```python
from build123d import *

# Parameters (mm, degrees)
F1_DEPTH = 25
F2_DEPTH = 25
F3_DEPTH = 25
F4_DEPTH = 25
F5_DEPTH = 25
F6_DEPTH = 25


with BuildPart() as f1:
    # F0 (on Top) → F1 (new body)
    with BuildSketch(Plane.XY):
        Polygon((264.877629, 90.833528), (-135.122371, 90.833528), (-18.141241, -204.166472), (181.858759, -204.166472), align=None)
    extrude(amount=F1_DEPTH)

    # F0 (on Top) → F2 (join)
    with BuildSketch(Plane.XY):
        Polygon((264.877629, 90.833528), (-135.122371, 90.833528), (-18.141241, -204.166472), (181.858759, -204.166472), align=None)
    extrude(amount=F2_DEPTH)

    # F0 (on Top) → F3 (join)
    with BuildSketch(Plane.XY):
        Polygon((264.877629, 90.833528), (-135.122371, 90.833528), (-18.141241, -204.166472), (181.858759, -204.166472), align=None)
    extrude(amount=F3_DEPTH)

    # F0 (on Top) → F4 (join)
    with BuildSketch(Plane.XY):
        Polygon((264.877629, 90.833528), (-135.122371, 90.833528), (-18.141241, -204.166472), (181.858759, -204.166472), align=None)
    extrude(amount=F4_DEPTH)

    # F0 (on Top) → F5 (join)
    with BuildSketch(Plane.XY):
        Polygon((264.877629, 90.833528), (-135.122371, 90.833528), (-18.141241, -204.166472), (181.858759, -204.166472), align=None)
    extrude(amount=F5_DEPTH)

    # F0 (on Top) → F6 (join)
    with BuildSketch(Plane.XY):
        Polygon((264.877629, 90.833528), (-135.122371, 90.833528), (-18.141241, -204.166472), (181.858759, -204.166472), align=None)
    extrude(amount=F6_DEPTH)


solid = f1.part
```
Here's how the part is built. I have some questions about the finished solid (model axes, mm). Round coordinates to 2 decimals unless told otherwise and drop trailing zeros. Loops run counter-clockwise (first coordinate to the right, second up) from the corner with the lowest first, then second, coordinate; pieces in that order, holes last.
1. If I drill on probe 1 along X at (y, z) = (-166.5, 6.75); probe 2 along X at (y, z) = (-31, 8), over which ranges is the centre line in solid material (lowest first)?
Answers:
probe 1: x = -33.08 to 192.46
probe 2: x = -86.81 to 230.59
2. Will these pins go through, and if not, where does the flat tip stop? pin 1 (6 mm diameter, centred on y = 58, z = 16.5, fed in from +X); pin 2 (8 mm diameter, centred on y = 14, z = 12.5, fed in from +X); pin 3 (8 mm diameter, centred on y = -69, z = 15, fed in from +X).
Answers:
pin 1: stops at x = 256.48
pin 2: stops at x = 244.38
pin 3: stops at x = 221.02
3. Suppose I cut it at B-B, the plane y = 36.5. Please give me the cut outline in (x, z).
Answers:
outline: (-113.58, 0) - (249.59, 0) - (249.59, 25) - (-113.58, 25) - close
4. Suppose I cut it at A-A, the plane z = 5.75. Please give me the cut outline in (x, y).
Answers:
outline: (-135.12, 90.83) - (-18.14, -204.17) - (181.86, -204.17) - (264.88, 90.83) - close
